Here's how the part is built. I have some questions about the finished solid (model axes, mm). A direction names the side the tool comes from. Round coordinates to 2 decimals unless told otherwise and drop trailing zeros. Loops run counter-clockwise (first coordinate to the right, second up) from the corner with the lowest first, then second, coordinate; pieces in that order, holes last. Notation, with made-up numbers: (16, 63) - (54, 63) arc R30 ccw to (54, 94) - close; hole circle Ø3 at (-36, 20.25). An arc over 180 degrees is marked (long way). Answer as a JSON object with one key per item and string values. Group by question number.
1) Will these pins go through, and if not, where does the flat tip stop? P1, Ø5, axis at x = 7, y = 5.5, coming from the -Z side; P2, Ø1.7, axis at x = 0, z = 39.9, coming from the -Y side; P3, Ø1.5, axis at x = -2.5, z = 63, coming from the -Y side; P4, Ø3, axis at x = -0.5, z = 17, coming from the +Y side.
2) I want a section at B-B, the plane x = -7. Please give me the cut outline in (y, z).
3) If we mould it in two halves opening along X, with no side actions, what happens to faces 5 (the face through (0, -4, 121.6)), 6 (the face through (-1.172, 8.923, 120.079)), 7 (the face through (0, 0, 112.6))? For each: pulls with the +X half, pulls with the -X half, needs draft (parallel to the pull), parting line crosses it, or undercut.
4) I want a section at C-C, the plane z = 106.5. Please give me the cut outline in (x, y).
5) I want a section at A-A, the plane y = -7.25. Please give me the cut outline in (x, z), then the cut area to 3 significant figures.
6) Which directions (+Z, -Z, +X, -X, +Y, -Y) give clear straight access to the entire face, cutting with the end or side of a thin tool? Please do faces 1 (the face through (-3, 0, 117)), 2 (the face through (2, -6, 110.6)), 3 (the face through (-1.172, 8.923, 106.595)), 4 (the face through (-0.867, -3.905, 100.317)).
7) I want a section at D-D, the plane z = 39.9. Please give me the cut outline in (x, y).
8) If I drill on line 1 along Y through (x, z) = (0, 114.75); line 2 along Z through (x, y) = (0, -2.3); line 3 along Z through (x, y) = (7, 2.75), over which ranges is the centre line in solid material (lowest first)? Write a range as [from, to].
from build123d import *

# Parameters (mm, degrees)
SKETCH1_R               = 3
BOSS_EXTRUDE1_DEPTH     = 98
SKETCH2_R               = 4
BOSS_EXTRUDE2_DEPTH     = 4.7
SKETCH3_R               = 9
BOSS_EXTRUDE3_DEPTH     = 7.9
SKETCH4_R               = 5.9
BOSS_EXTRUDE4_DEPTH     = 8
SKETCH5_R               = 9
BOSS_EXTRUDE5_DEPTH     = 3
SKETCH6_R               = 1.4
CUT_EXTRUDE1_DEPTH      = 82
CUT_EXTRUDE1_DEPTH_BACK = 82
SKETCH7_R               = 3
SKETCH7_R_2             = 0.75
CUT_EXTRUDE2_DEPTH      = 9


with BuildPart() as part:
    # Sketch1 → Boss-Extrude1 (new body)
    with BuildSketch(Plane.XY):
        Circle(SKETCH1_R)
    extrude(amount=BOSS_EXTRUDE1_DEPTH)

    # Sketch2 → Boss-Extrude2 (add)
    with BuildSketch(Plane.XY.offset(98)):
        Circle(SKETCH2_R)
    extrude(amount=BOSS_EXTRUDE2_DEPTH)

    # Sketch3 → Boss-Extrude3 (add)
    with BuildSketch(Plane.XY.offset(102.7)):
        Circle(SKETCH3_R)
    extrude(amount=BOSS_EXTRUDE3_DEPTH)

    # Sketch4 → Boss-Extrude4 (add)
    with BuildSketch(Plane.XY.offset(110.6)):
        Circle(SKETCH4_R)
    extrude(amount=BOSS_EXTRUDE4_DEPTH)

    # Sketch5 → Boss-Extrude5 (add)
    with BuildSketch(Plane.XY.offset(118.6)):
        Circle(SKETCH5_R)
    extrude(amount=BOSS_EXTRUDE5_DEPTH)

    # Sketch6 → Cut-Extrude1 (cut, two sides)
    with BuildSketch(Plane(origin=(0, 0, 0), x_dir=(1, 0, 0), z_dir=(0, 1, 0))) as cut_extrude1_sk:
        with Locations((0, -39.9)):
            Circle(SKETCH6_R)
    extrude(amount=CUT_EXTRUDE1_DEPTH, mode=Mode.SUBTRACT)
    extrude(cut_extrude1_sk.sketch, amount=-CUT_EXTRUDE1_DEPTH_BACK, mode=Mode.SUBTRACT)

    # Sketch7 → Cut-Extrude2 (cut)
    with BuildSketch(Plane.XY.offset(121.6)):
        Circle(SKETCH7_R)
        with Locations((1.637751338, 7.588247864)):
            Circle(SKETCH7_R_2)
    extrude(amount=-CUT_EXTRUDE2_DEPTH, mode=Mode.SUBTRACT)


solid = part.part
Outcome:
{
 "1": {"P1": "z = 102.7", "P2": "through", "P3": "y = -2.44", "P4": "y = 3"},
 "2": {"outline": "(-5.66, 102.7) - (5.66, 102.7) - (5.66, 110.6) - (-5.66, 110.6) - close; (-5.66, 118.6) - (5.66, 118.6) - (5.66, 121.6) - (-5.66, 121.6) - close"},
 "3": {"face 5": "needs draft", "face 6": "parting line crosses it", "face 7": "undercut"},
 "4": {"outline": "circle Ø18 at (0, 0)"},
 "5": {"outline": "(-5.33, 102.7) - (5.33, 102.7) - (5.33, 110.6) - (-5.33, 110.6) - close; (-5.33, 118.6) - (5.33, 118.6) - (5.33, 121.6) - (-5.33, 121.6) - close", "area": "116 mm^2"},
 "6": {"face 1": "+Z", "face 2": "none", "face 3": "+Z, -Z", "face 4": "-Z"},
 "7": {"outline": "(-1.4, -2.65) - (-1.4, 2.65) arc R3 ccw to start; (1.4, -2.65) arc R3 ccw to (1.4, 2.65) - close"},
 "8": {"line 1": "[-5.9, -3], [3, 5.9]", "line 2": "[0, 38.5], [41.3, 112.6]", "line 3": "[102.7, 110.6], [118.6, 121.6]"}
}
